Verification items for the finished model (mm, model axes). Give positions to 0.01 mm unless a question says otherwise; leave off trailing zeros. Write each loop counter-clockwise with the first axis right and the second up, starting at its lowest first coordinate (ties: lowest second). Pieces come first, ordered by that corner, then holes. Notation, with made-up numbers: (11.5, 63) - (56.5, 63) arc R13 ccw to (56.5, 80) - close; hole circle Ø5 at (85.5, 57.5). An arc over 180 degrees is marked (long way). Put each result on its own line as item: value.
from build123d import *

# Parameters (mm, degrees)
SKETCH_1_W          = 186
SKETCH_1_H          = 20
EXTRUDE_1_DEPTH     = 14
SKETCH_2_W          = 186
SKETCH_2_H          = 20
CUT_EXTRUDE_2_DEPTH = 2
SKETCH_3_W          = 177
SKETCH_3_H          = 11
CUT_EXTRUDE_3_DEPTH = 4
SKETCH_4_R          = 2.75
CUT_EXTRUDE_6_DEPTH = 5.5
SKETCH_5_W          = 185.880265185
SKETCH_5_H          = 100
EXTRUDE_2_DEPTH     = 5.5
FILLET_1_R          = 10
FILLET_2_R          = 10
FILLET_3_R          = 10
FILLET_4_R          = 10
FILLET_6_R          = 2
FILLET_7_R          = 2
FILLET_8_R          = 2
FILLET_9_R          = 2


with BuildPart() as part:
    # 草图1 → 凸台-拉伸1 (new body)
    with BuildSketch(Plane(origin=(0, 0, 0), x_dir=(1, 0, 0), z_dir=(0, 1, 0))):
        Rectangle(SKETCH_1_W, SKETCH_1_H)
    extrude(amount=EXTRUDE_1_DEPTH)

    # 草图2 → 切除-拉伸2 (cut)
    with BuildSketch(Plane(origin=(0, 14, 0), x_dir=(1, 0, 0), z_dir=(0, 1, 0))):
        Rectangle(SKETCH_2_W, SKETCH_2_H)
    extrude(amount=-CUT_EXTRUDE_2_DEPTH, mode=Mode.SUBTRACT)

    # 草图3 → 切除-拉伸3 (cut)
    with BuildSketch(Plane.XZ):
        Rectangle(SKETCH_3_W, SKETCH_3_H)
    extrude(amount=-CUT_EXTRUDE_3_DEPTH, mode=Mode.SUBTRACT)

    # 草图4 → 切除-拉伸6 (cut)
    with BuildSketch(Plane.XZ.offset(-4)):
        with Locations(Location((-72, 0, 0), (0, 0, 270))):
            Circle(SKETCH_4_R)
        with Locations(Location((-38, 0, 0), (0, 0, 270))):
            Circle(SKETCH_4_R)
        with Locations(Location((38, 0, 0), (0, 0, 270))):
            Circle(SKETCH_4_R)
        with Locations(Location((72, 0, 0), (0, 0, 270))):
            Circle(SKETCH_4_R)
    extrude(amount=-CUT_EXTRUDE_6_DEPTH, mode=Mode.SUBTRACT)

    # 草图5 → 凸台-拉伸2 (add)
    with BuildSketch(Plane(origin=(0, 12, 0), x_dir=(1, 0, 0), z_dir=(0, 1, 0))):
        with Locations((0.140286992, 0)):
            Rectangle(SKETCH_5_W, SKETCH_5_H)
    extrude(amount=EXTRUDE_2_DEPTH)

    # 圆角1
    fillet_1_edges = [part.edges().sort_by_distance(p)[0] for p in [
        (-92.7998456, 14.75, 50),
    ]]
    fillet(fillet_1_edges, radius=FILLET_1_R)

    # 圆角2
    fillet_2_edges = [part.edges().sort_by_distance(p)[0] for p in [
        (93.080419585, 14.75, 50),
    ]]
    fillet(fillet_2_edges, radius=FILLET_2_R)

    # 圆角3
    fillet_3_edges = [part.edges().sort_by_distance(p)[0] for p in [
        (93.080419585, 14.75, -50),
    ]]
    fillet(fillet_3_edges, radius=FILLET_3_R)

    # 圆角4
    fillet_4_edges = [part.edges().sort_by_distance(p)[0] for p in [
        (-92.7998456, 14.75, -50),
    ]]
    fillet(fillet_4_edges, radius=FILLET_4_R)

    # 圆角6
    fillet_6_edges = [part.edges().sort_by_distance(p)[0] for p in [
        (0, 0, -10),
    ]]
    fillet(fillet_6_edges, radius=FILLET_6_R)

    # 圆角7
    fillet_7_edges = [part.edges().sort_by_distance(p)[0] for p in [
        (0, 0, 10),
    ]]
    fillet(fillet_7_edges, radius=FILLET_7_R)

    # 圆角8
    # the kernel refuses this fillet: 2 mm, written as the material it takes off along each edge
    with BuildSketch(Plane(origin=(-93, 0, 8), x_dir=(1, 0, 0), z_dir=(0, 0, -1))) as fillet_8_piece_1:
        with BuildLine():
            CenterArc((FILLET_8_R, -FILLET_8_R), FILLET_8_R, 90, 90)
            Line((0, -FILLET_8_R), (0, 0))
            Line((0, 0), (FILLET_8_R, 0))
        make_face()
    extrude(amount=16, mode=Mode.SUBTRACT)
    with BuildSketch(Plane(origin=(-93, 2, -8), x_dir=(0, 0, -1), z_dir=(0, 1, 0))) as fillet_8_piece_2:
        with BuildLine():
            CenterArc((2 - FILLET_8_R, -FILLET_8_R), FILLET_8_R, 0, 90)
            Line((2 - FILLET_8_R, 0), (2, 0))
            Line((2, 0), (2, -FILLET_8_R))
        make_face()
    revolve(axis=Axis((-93, 2, -8), (-1, 0, 0)), revolution_arc=90, mode=Mode.SUBTRACT)
    with BuildSketch(Plane(origin=(-93, 2, 8), x_dir=(0, -1, 0), z_dir=(0, 0, -1))) as fillet_8_piece_3:
        with BuildLine():
            CenterArc((2 - FILLET_8_R, -FILLET_8_R), FILLET_8_R, 0, 90)
            Line((2 - FILLET_8_R, 0), (2, 0))
            Line((2, 0), (2, -FILLET_8_R))
        make_face()
    revolve(axis=Axis((-93, 2, 8), (-1, 0, 0)), revolution_arc=90, mode=Mode.SUBTRACT)
    with BuildSketch(Plane(origin=(-93, 2, 10), x_dir=(1, 0, 0), z_dir=(0, 1, 0))) as fillet_8_piece_4:
        with BuildLine():
            CenterArc((FILLET_8_R, FILLET_8_R), FILLET_8_R, 180, 90)
            Line((0, FILLET_8_R), (0, 0))
            Line((0, 0), (FILLET_8_R, 0))
        make_face()
    extrude(amount=10, mode=Mode.SUBTRACT)
    with BuildSketch(Plane(origin=(-93, 2, -10), x_dir=(1, 0, 0), z_dir=(0, 1, 0))) as fillet_8_piece_5:
        with BuildLine():
            CenterArc((FILLET_8_R, -FILLET_8_R), FILLET_8_R, 90, 90)
            Line((0, -FILLET_8_R), (0, 0))
            Line((0, 0), (FILLET_8_R, 0))
        make_face()
    extrude(amount=10, mode=Mode.SUBTRACT)

    # 圆角9
    fillet_9_edges = [part.edges().sort_by_distance(p)[0] for p in [
        (93, 0, 0),
        (93, 0.585786438, -9.414213562),
        (93, 0.585786438, 9.414213562),
        (93, 7, -10),
        (93, 7, 10),
    ]]
    fillet(fillet_9_edges, radius=FILLET_9_R)


solid = part.part
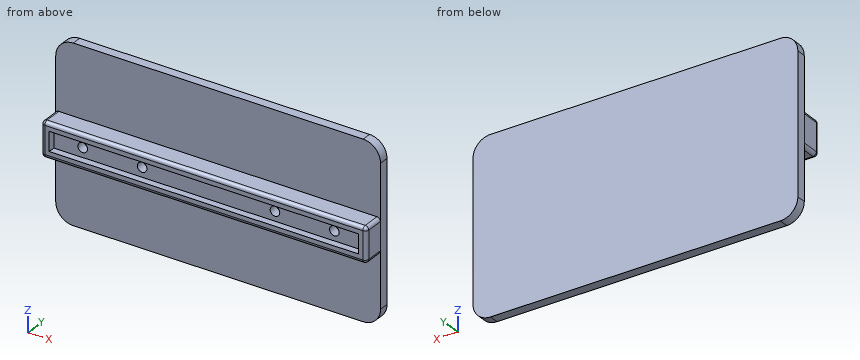
Q1. Scan lines: line 1 along X through (y, z) = (7, 0); line 2 along Z through (x, y) = (6, 1.75); line 3 along X through (y, z) = (8, -6.5). Record each from-to range of solid material in increasing order.
Answers follow:
line 1: x = -93 to -74.75, -69.25 to -40.75, -35.25 to 35.25, 40.75 to 69.25, 74.75 to 93
line 2: z = -9.98 to -5.5, 5.5 to 9.98
line 3: x = -93 to 93
Q2. Section check A-A, the plane x = -16. Record the cut outline in (y, z), plus the area to 3 significant figures.
Answers follow:
outline: (0, -8) arc R2 ccw to (2, -10) - (12, -10) - (12, -50) - (17.5, -50) - (17.5, 50) - (12, 50) - (12, 10) - (2, 10) arc R2 ccw to (0, 8) - (0, 5.5) - (4, 5.5) - (4, -5.5) - (0, -5.5) - close
area: 744 mm2
Q3. Section check D-D, the plane z = -15. Record the cut outline in (x, y), plus the area to 3 significant figures.
Answers follow:
outline: (-92.8, 12) - (93.08, 12) - (93.08, 17.5) - (-92.8, 17.5) - close
area: 1,020 mm2
Q4. Section check C-C, the plane x = 72. Record the cut outline in (y, z).
Answers follow:
outline: (0, -8) arc R2 ccw to (2, -10) - (12, -10) - (12, -50) - (17.5, -50) - (17.5, 50) - (12, 50) - (12, 10) - (2, 10) arc R2 ccw to (0, 8) - (0, 5.5) - (4, 5.5) - (4, 2.75) - (9.5, 2.75) - (9.5, -2.75) - (4, -2.75) - (4, -5.5) - (0, -5.5) - close
Q5. Go/stop test with flat-tipped pins: pin 1 Ø4.5 at (x, y) = (43.5, 1.5) entering from +Z; pin 2 Ø4.5 at (x, z) = (-38, 0) entering from -Y; pin 3 Ø1.2 at (y, z) = (2.5, 1) entering from +X. Record where each tip stops, or that it passes through.
Answers follow:
pin 1: stops at z = 10
pin 2: stops at y = 9.5
pin 3: stops at x = 93
